The model under review builds one solid part; all positions refer to its coordinate system, in mm. Give positions to 0.01 mm unless a question says otherwise; leave off trailing zeros. Put each result on its own line as item: value.
```python
from build123d import *

# Parameters (mm, degrees)
SKETCH1_4_W         = 263.6
SKETCH1_4_H         = 20
SKETCH1_4_R         = 2
BOSS_EXTRUDE3_DEPTH = 5


with BuildPart() as part:
    # Sketch1_4 → Boss-Extrude3 (new body)
    with BuildSketch(Plane(origin=(0, 0, 0), x_dir=(1, 0, 0), z_dir=(0, 1, 0))):
        Rectangle(SKETCH1_4_W, SKETCH1_4_H)
        with Locations(Location((-120, 0, 0), (0, 0, 270))):
            Circle(SKETCH1_4_R, mode=Mode.SUBTRACT)
        with Locations(Location((0, 0, 0), (0, 0, 270))):
            Circle(SKETCH1_4_R, mode=Mode.SUBTRACT)
        with Locations(Location((120, 0, 0), (0, 0, 270))):
            Circle(SKETCH1_4_R, mode=Mode.SUBTRACT)
    extrude(amount=BOSS_EXTRUDE3_DEPTH)


solid = part.part
```
(1) The part is to be moulded in two halves that separate along X. For faces 1 (the flat face through (-2, 2, -10)), 2 (the flat face through (-131.8, 2, 0)), 3 (the cylindrical face through (-118.314, 2.465, 1.075)), say which applies: pulls with the +X half, pulls with the -X half, needs draft (parallel to the pull), parting line crosses it, or undercut.
The answers:
face 1: needs draft
face 2: pulls with the -X half
face 3: undercut
(2) Clearance check with a flat-ended pin moving along its axis: pin 1 Ø3 at (x, z) = (-120, 0) entering from -Y. State where the tip first meets the part, or that it passes through.
The answers:
pin 1: through
(3) Wall thickness on L1, parallel to X at y = 1, z = 0; L2, parallel to X at y = 4.5, z = 1.75: over which ranges is each line inside the solid? List them lowest first.
The answers:
L1: -131.8 to -122, -118 to -2, 2 to 118, 122 to 131.8
L2: -131.8 to -120.97, -119.03 to -0.97, 0.97 to 119.03, 120.97 to 131.8
